Read the model definition and answer for the solid it produces. Units are mm, in the model's axes. Give positions to 0.01 mm unless a question says otherwise; leave off trailing zeros. Order: outer loops, then holes, each group sorted by start corner. A loop starts at its lowest first (then second) coordinate and runs counter-clockwise, first axis right, second up.
Item 1: A cutting plane is placed at A-A (z = 2). Write down the section's boundary in (x, y), plus the area to 3 significant figures.
Item 2: Given pin 1 Ø2.5 at (x, y) = (-5.5, 5.5) entering from -Z, flat-ended and moving along its own axis, determine where the tip first touches the part or whether it passes through.
Item 3: A cutting plane is placed at B-B (y = 5.5). Write down the section's boundary in (x, z).
Item 4: Find the intervals of material crossed by line 1 along Y through (x, z) = (-5.5, 5.75); line 2 along X through (y, z) = (6.5, 1.5); line 3 along Y through (x, z) = (5, 5.5), in increasing order.
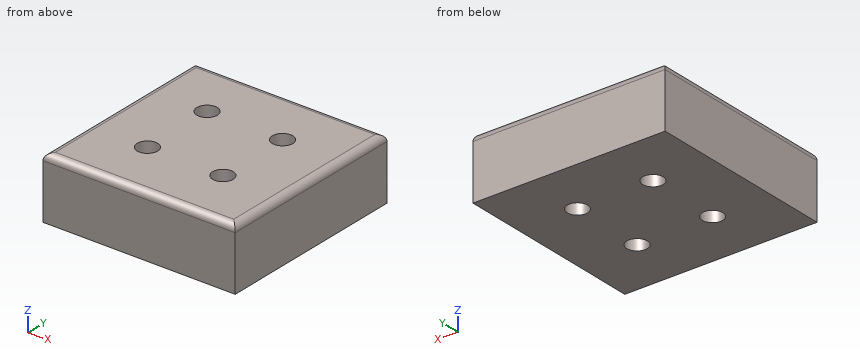
from build123d import *

# Parameters (mm, degrees)
F0_W     = 28
F0_H     = 28
F1_DEPTH = 9
F3_D     = 3
F4_R     = 1


# Not quite as in the source:
# - a feature names something its author has since deleted; it is built from what else it names


with BuildPart() as f1:
    # F0 (on Top) → F1 (new body)
    with BuildSketch(Plane.XY):
        Rectangle(F0_W, F0_H)
    extrude(amount=F1_DEPTH)

    # F3 (through all)
    with Locations(Plane.XY.offset(9)):
        with Locations((5.5, 5.5), (-5.5, 5.5), (-5.5, -5.5), (5.5, -5.5)):
            Hole(F3_D / 2)

    # F4
    f4_edges = [f1.edges().sort_by_distance(p)[0] for p in [
        (0, 14, 9),
        (-14, 0, 9),
        (0, -14, 9),
        (14, 0, 9),
    ]]
    fillet(f4_edges, radius=F4_R)


solid = f1.part
Response values:
1. outline: (-14, -14) - (14, -14) - (14, 14) - (-14, 14) - close; hole circle Ø3 at (-5.5, -5.5); hole circle Ø3 at (-5.5, 5.5); hole circle Ø3 at (5.5, -5.5); hole circle Ø3 at (5.5, 5.5)
1. area: 756 mm2
2. pin 1: passes through
3. outline: (-14, 0) - (-7, 0) - (-7, 9) - (-13, 9) arc R1 ccw to (-14, 8) - close; (-4, 0) - (4, 0) - (4, 9) - (-4, 9) - close; (7, 0) - (14, 0) - (14, 8) arc R1 ccw to (13, 9) - (7, 9) - close
4. line 1: y = -14 to -7, -4 to 4, 7 to 14
4. line 2: x = -14 to -6.62, -4.38 to 4.38, 6.62 to 14
4. line 3: y = -14 to -6.91, -4.09 to 4.09, 6.91 to 14
